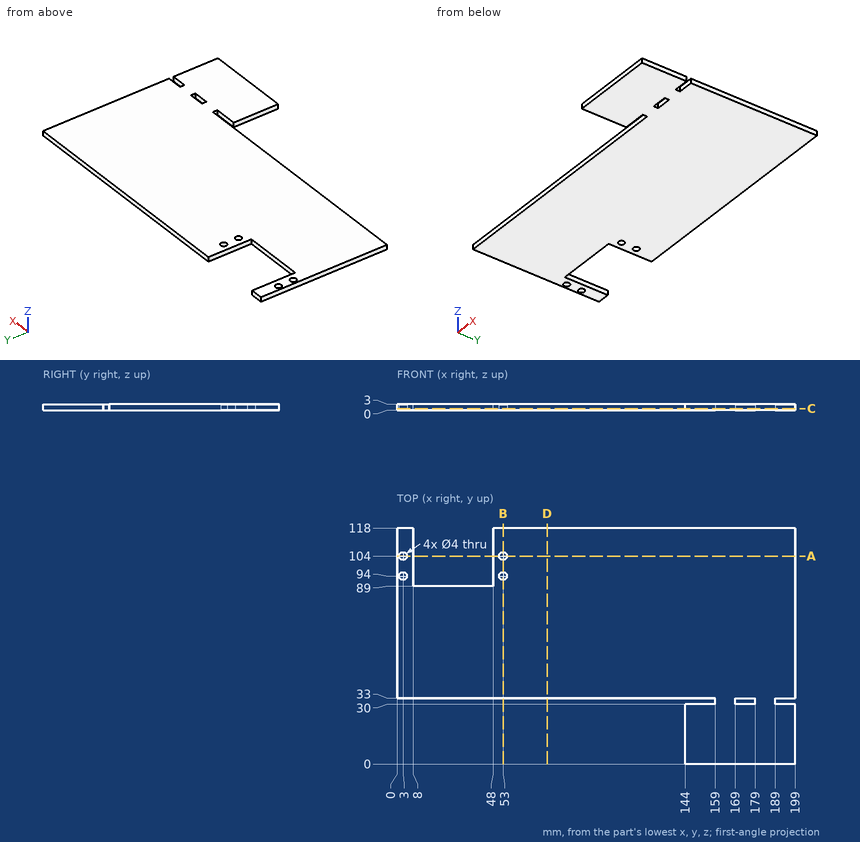
Geometry: see drawing. Coordinates: mm, zero at the bounding-box minimum. Round coordinates to 2 decimals unless told otherwise and drop trailing zeros. Order: outer loops, then holes, each group sorted by start corner. A loop starts at its lowest first (then second) coordinate and runs counter-clockwise, first axis right, second up. Notation, with made-up numbers: (75.5, 47) - (79.5, 47) arc R28 cw to (79.5, 66) - close; hole circle Ø1 at (-12.75, 68). An arc over 180 degrees is marked (long way). One line per question, with ' | ' between items. Start each with the question number.
1) Contact query for flat-ended pins moving along their axis: P1, Ø6.5, axis at x = 53, y = 104, coming from the -Z side; P2, Ø1.5, axis at y = 31.5, z = 1, coming from the +X side; P3, Ø1.5, axis at y = 31.5, z = 2, coming from the -X side. Output: stop coordinate, or through.
2) Cut plane D-D, the plane x = 75. Return the cut outline in (y, z), then the cut area to 3 significant figures.
3) Ray query, probe 1 along Y at (x, z) = (53, 2.1); probe 2 along X at (y, z) = (104, 1.95); probe 3 along X at (y, z) = (108, 1.8). Return the intervals inside material, ascending.
4) Cut plane A-A, the plane y = 104. Return the cut outline in (x, z), then the cut area to 3 significant figures.
5) Cut plane C-C, the plane z = 0.75. Return the cut outline in (x, y).
6) Cut plane B-B, the plane x = 53. Return the cut outline in (y, z).
Worked out:
1) P1: stops at z = 0 | P2: stops at x = 189 | P3: stops at x = 159
2) outline: (33, 0) - (118, 0) - (118, 3) - (33, 3) - close | area: 255 mm^2
3) probe 1: y = 33 to 92, 96 to 102, 106 to 118 | probe 2: x = 0 to 1, 5 to 8, 48 to 51, 55 to 199 | probe 3: x = 0 to 8, 48 to 199
4) outline: (0, 0) - (1, 0) - (1, 3) - (0, 3) - close; (5, 0) - (8, 0) - (8, 3) - (5, 3) - close; (48, 0) - (51, 0) - (51, 3) - (48, 3) - close; (55, 0) - (199, 0) - (199, 3) - (55, 3) - close | area: 453 mm^2
5) outline: (0, 33) - (159, 33) - (159, 30) - (144, 30) - (144, 0) - (199, 0) - (199, 30) - (189, 30) - (189, 33) - (199, 33) - (199, 118) - (48, 118) - (48, 89) - (8, 89) - (8, 118) - (0, 118) - close; hole circle Ø4 at (3, 94); hole circle Ø4 at (3, 104); hole circle Ø4 at (53, 94); hole circle Ø4 at (53, 104); hole (169, 30) - (179, 30) - (179, 33) - (169, 33) - close
6) outline: (33, 0) - (92, 0) - (92, 3) - (33, 3) - close; (96, 0) - (102, 0) - (102, 3) - (96, 3) - close; (106, 0) - (118, 0) - (118, 3) - (106, 3) - close
